The model under review builds one solid part; all positions refer to its coordinate system, in mm. A direction names the side the tool comes from. Coordinates: 2 decimals unless noted, no trailing zeros. Order: outer loops, then holes, each group sorted by start corner. A loop starts at its lowest first (then second) coordinate and runs counter-clockwise, first axis right, second up.
```python
from build123d import *
from build123d.topology import SkipClean

# Parameters (mm, degrees)
BOSS_EXTRUDE1_DEPTH = 42.000000074
BOSS_EXTRUDE2_START = 2.000000064
BOSS_EXTRUDE2_DEPTH = 2.000000064
BOSS_EXTRUDE3_DEPTH = 15
BOSS_EXTRUDE4_DEPTH = 15
BOSS_EXTRUDE5_DEPTH = 15
BOSS_EXTRUDE6_DEPTH = 15
RIB1_START          = -1.27
RIB1_DEPTH          = 2.54
RIB2_START          = -1.27
RIB2_DEPTH          = 2.54
SKETCH18_W          = 2.54
SKETCH18_H          = 96.020000238
BOSS_EXTRUDE7_DEPTH = 15
SKETCH19_W          = 2.54
SKETCH19_H          = 96.020000238
BOSS_EXTRUDE8_DEPTH = 15


# Read off the part's stored shape, not the designer's step: Rib1, Rib2
with BuildPart() as part:
    # Sketch1 → Boss-Extrude1 (new body)
    with BuildSketch(Plane.ZY):
        with BuildLine():
            Line((-45.001214275, 0), (-42.443087035, 0))
            ThreePointArc((-42.443087035, 0), (25, 141.699999936), (92.443087035, 0))
            Line((92.443087035, 0), (95.001214275, 0))
            ThreePointArc((95.001214275, 0), (25, 143.7), (-45.001214275, 0))
        make_face()
    extrude(amount=-BOSS_EXTRUDE1_DEPTH)

    # Sketch2 → Boss-Extrude2 (add)
    with SkipClean():  # the faces are left unmerged after this step: merging them gives an invalid solid
        with BuildSketch(Plane.ZY.offset(BOSS_EXTRUDE2_START)):
            with BuildLine():
                Line((-160, 0), (-45.001214275, 0))
                ThreePointArc((-45.001214275, 0), (-63.9, 54.800000001), (-45.001214274, 109.600000001))
                Line((-45.001214275, 109.600000002), (-160, 109.600000002))
                Line((-160, 109.600000002), (-162.000000064, 109.600000002))
                Line((-162.000000064, 109.600000002), (-162.000000064, 0))
                Line((-162.000000064, 0), (-160, 0))
            make_face()
            with BuildLine():
                ThreePointArc((-45.001214275, 0), (25, 143.7), (95.001214275, 0))
                Line((95.001214275, 0), (92.443087035, 0))
                ThreePointArc((92.443087035, 0), (25, 141.699999936), (-42.443087035, 0))
                Line((-42.443087035, 0), (-45.001214275, 0))
            make_face()
            with BuildLine():
                ThreePointArc((95.001214275, 109.6), (113.9, 54.8), (95.001214275, 0))
                Line((95.001214275, 0), (120, 0))
                Line((120, 0), (122.000000064, 0))
                Line((122.000000064, 0), (122.000000064, 109.6))
                Line((122.000000064, 109.6), (120, 109.6))
                Line((120, 109.6), (95.001214275, 109.6))
            make_face()
        extrude(amount=-BOSS_EXTRUDE2_DEPTH)

    # Sketch7 → Boss-Extrude3 (add)
    with SkipClean():  # the faces are left unmerged after this step: merging them gives an invalid solid
        with BuildSketch(Plane(origin=(0, 0, 0), x_dir=(0, 0, -1), z_dir=(1, 0, 0))):
            with BuildLine():
                Line((49.821453399, 6.789999882), (162.000000064, 6.789999882))
                Line((162.000000064, 6.789999882), (162.000000064, 4.249999882))
                Line((162.000000064, 4.249999882), (48.129388676, 4.249999882))
                ThreePointArc((48.129388676, 4.249999882), (48.986321828, 5.512738133), (49.821453399, 6.789999882))
            make_face()
        extrude(amount=BOSS_EXTRUDE3_DEPTH)

    # Sketch10 → Boss-Extrude4 (add)
    with SkipClean():  # the faces are left unmerged after this step: merging them gives an invalid solid
        with BuildSketch(Plane(origin=(0, 0, 0), x_dir=(0, 0, -1), z_dir=(1, 0, 0))):
            with BuildLine():
                Line((-99.821453399, 6.789999882), (-122.000000064, 6.789999882))
                Line((-122.000000064, 6.789999882), (-122.000000064, 4.249999882))
                Line((-122.000000064, 4.249999882), (-98.129388676, 4.249999882))
                ThreePointArc((-98.129388676, 4.249999882), (-98.986321828, 5.512738133), (-99.821453399, 6.789999882))
            make_face()
        extrude(amount=BOSS_EXTRUDE4_DEPTH)

    # Sketch12 → Boss-Extrude5 (add)
    with SkipClean():  # the faces are left unmerged after this step: merging them gives an invalid solid
        with BuildSketch(Plane(origin=(0, 0, 0), x_dir=(0, 0, -1), z_dir=(1, 0, 0))):
            with BuildLine():
                Line((-122.000000064, 105.35000012), (-98.129388674, 105.35000012))
                ThreePointArc((-98.129388674, 105.35000012), (-98.986321827, 104.087261869), (-99.821453397, 102.81000012))
                Line((-99.821453397, 102.81000012), (-122.000000064, 102.81000012))
                Line((-122.000000064, 102.81000012), (-122.000000064, 105.35000012))
            make_face()
        extrude(amount=BOSS_EXTRUDE5_DEPTH)

    # Sketch14 → Boss-Extrude6 (add)
    with SkipClean():  # the faces are left unmerged after this step: merging them gives an invalid solid
        with BuildSketch(Plane(origin=(0, 0, 0), x_dir=(0, 0, -1), z_dir=(1, 0, 0))):
            with BuildLine():
                Line((162.000000064, 105.35000012), (48.129388674, 105.35000012))
                ThreePointArc((48.129388674, 105.35000012), (48.986321827, 104.087261869), (49.821453397, 102.81000012))
                Line((49.821453397, 102.81000012), (162.000000064, 102.81000012))
                Line((162.000000064, 102.81000012), (162.000000064, 105.35000012))
            make_face()
        extrude(amount=BOSS_EXTRUDE6_DEPTH)

    # Rib1 outline → Rib1 (add)
    with SkipClean():  # the faces are left unmerged after this step: merging them gives an invalid solid
        with BuildSketch(Plane(origin=(0, 0, -111.200000064), x_dir=(-1, 0, 0), z_dir=(0, 0, -1)).offset(RIB1_START)):
            Polygon((0, 102.81000012), (-15, 102.81000012), (0, 54.800000001), align=None)
        extrude(amount=RIB1_DEPTH)

    # Rib2 outline → Rib2 (add)
    with SkipClean():  # the faces are left unmerged after this step: merging them gives an invalid solid
        with BuildSketch(Plane(origin=(0, 0, -111.200000064), x_dir=(-1, 0, 0), z_dir=(0, 0, -1)).offset(RIB2_START)):
            Polygon((0, 54.800000001), (-15, 6.789999882), (0, 6.789999882), align=None)
        extrude(amount=RIB2_DEPTH)

    # Sketch18 → Boss-Extrude7 (add)
    with SkipClean():  # the faces are left unmerged after this step: merging them gives an invalid solid
        with BuildSketch(Plane(origin=(0, 0, 0), x_dir=(0, 0, -1), z_dir=(1, 0, 0))):
            with Locations((160.730000064, 54.800000001)):
                Rectangle(SKETCH18_W, SKETCH18_H)
        extrude(amount=BOSS_EXTRUDE7_DEPTH)

    # Sketch19 → Boss-Extrude8 (add)
    with SkipClean():  # the faces are left unmerged after this step: merging them gives an invalid solid
        with BuildSketch(Plane(origin=(0, 0, 0), x_dir=(0, 0, -1), z_dir=(1, 0, 0))):
            with Locations((-120.730000064, 54.800000001)):
                Rectangle(SKETCH19_W, SKETCH19_H)
        extrude(amount=BOSS_EXTRUDE8_DEPTH)


solid = part.part
```
(1) We need section C-C, the plane z = -98. Write out the cut boundary in (x, y), and give its area (3 significant figures).
A:
outline: (-2, 0) - (0, 0) - (0, 4.25) - (15, 4.25) - (15, 6.79) - (0, 6.79) - (0, 102.81) - (15, 102.81) - (15, 105.35) - (0, 105.35) - (0, 109.6) - (-2, 109.6) - close
area: 295 mm2
(2) Machinability: for faces 3 (the face through (7, 4.25, 110)), 4 (the face through (4, 20, -109.93)), 5 (the face through (7, 105.35, -106)), 6 (the face through (7, 4.25, -106)), which of the approach directions +Z, -Z, +X, -X, +Y, -Y give a long, thin tool a straight path to every point of the face, cutting with its end or side? Answer none if there is none.
A:
face 3: +Z, +X, -Y
face 4: +X
face 5: -Z, +X, +Y
face 6: -Z, +X, -Y
(3) Draft analysis for pull direction Z (two halves, no side actions). For faces 1 (the face through (7, 105.35, 110)), 2 (the face through (7.605, 79.141, -111.182)), state which applies: released by +Z, released by -Z, zero draft, split by the parting line, or undercut.
A:
face 1: zero draft
face 2: undercut
(4) We need section D-D, the plane y = 118. Write out the cut boundary in (x, z), and give its area (3 significant figures).
A:
outline: (-2, -37.52) - (42, -37.52) - (42, -34.64) - (-2, -34.64) - close; (-2, 84.64) - (42, 84.64) - (42, 87.52) - (-2, 87.52) - close
area: 253 mm2
(5) We need section B-B, the plane x = 9. Write out the cut boundary in (y, z).
A:
outline: (0, -45) arc R88.9 ccw to (4.25, -48.13) - (4.25, -162) - (105.35, -162) - (105.35, -48.13) arc R88.9 ccw to (105.35, 98.13) - (105.35, 122) - (4.25, 122) - (4.25, 98.13) arc R88.9 ccw to (0, 95) - (0, 92.44) arc R86.9 cw (long way) to (0, -42.44) - close; hole (6.79, -159.46) - (102.81, -159.46) - (102.81, -112.47) - (83.61, -112.47) - (83.61, -109.93) - (102.81, -109.93) - (102.81, -49.82) arc R88.9 cw to (6.79, -49.82) - (6.79, -109.93) - (25.99, -109.93) - (25.99, -112.47) - (6.79, -112.47) - close; hole (6.79, 99.82) arc R88.9 cw to (102.81, 99.82) - (102.81, 119.46) - (6.79, 119.46) - close
(6) For pin 1 Ø0.8 at (y, z) = (104, -133) entering from +X; pin 2 Ø1.3 at (y, z) = (3, 107) entering from +X; pin 3 Ø16.5 at (x, z) = (8.5, 107.5) entering from -Y, all flat-tipped, find the tip position at first contact; note any pin that passes through.
A:
pin 1: stops at x = 15
pin 2: stops at x = 0
pin 3: stops at y = 4.25
(7) Wall thickness on probe 1 along Z at (x, y) = (9.5, 54.8); probe 2 along Z at (x, y) = (26, 54.8); probe 3 along Y at (x, z) = (27, 25): over which ranges is each line inside the solid? List them lowest first.
A:
probe 1: z = -162 to -159.46, -63.9 to -61.9, 111.9 to 113.9, 119.46 to 122
probe 2: z = -63.9 to -61.9, 111.9 to 113.9
probe 3: y = 141.7 to 143.7
(8) We need section A-A, the plane y = 46. Write out the cut boundary in (x, z).
A:
outline: (-2, -162) - (15, -162) - (15, -159.46) - (0, -159.46) - (0, -112.47) - (2.75, -112.47) - (2.75, -109.93) - (0, -109.93) - (0, -63.46) - (42, -63.46) - (42, -61.45) - (-2, -61.45) - close; (-2, 111.45) - (42, 111.45) - (42, 113.46) - (0, 113.46) - (0, 119.46) - (15, 119.46) - (15, 122) - (-2, 122) - close
